from build123d import *

# Parameters (mm, degrees)
SKETCH1_R           = 15.75
SKETCH1_R_2         = 2
BOSS_EXTRUDE3_DEPTH = 10
SKETCH2_R           = 19.5
CUT_EXTRUDE1_DEPTH  = 10
CUT_EXTRUDE2_DEPTH  = 10
CUT_EXTRUDE3_DEPTH  = 10


with BuildPart() as part:
    # Sketch1 → Boss-Extrude3 (new body)
    with BuildSketch(Plane(origin=(0, 0, 0), x_dir=(1, 0, 0), z_dir=(0, 1, 0))):
        with BuildLine():
            Line((-52.326392464, -141.880675109), (47.673607536, -141.880675109))
            Line((47.673607536, -141.880675109), (47.673607536, 8.119324891))
            ThreePointArc((47.673607536, 8.119324891), (-2.326392464, 58.119324891), (-52.326392464, 8.119324891))
            Line((-52.326392464, 8.119324891), (-52.326392464, -141.880675109))
        make_face()
        with Locations((-2.326392464, 8.119324891)):
            Circle(SKETCH1_R, mode=Mode.SUBTRACT)
        with Locations((21.173607536, 8.119324891)):
            Circle(SKETCH1_R_2, mode=Mode.SUBTRACT)
        with Locations((9.423607536, -12.232272098)):
            Circle(SKETCH1_R_2, mode=Mode.SUBTRACT)
        with Locations((-14.076392464, -12.232272098)):
            Circle(SKETCH1_R_2, mode=Mode.SUBTRACT)
        with Locations((-25.826392464, 8.119324891)):
            Circle(SKETCH1_R_2, mode=Mode.SUBTRACT)
        with Locations((-14.076392464, 28.47092188)):
            Circle(SKETCH1_R_2, mode=Mode.SUBTRACT)
        with Locations((9.423607536, 28.47092188)):
            Circle(SKETCH1_R_2, mode=Mode.SUBTRACT)
        with Locations((-47.326392464, -116.880675109)):
            Circle(SKETCH1_R_2, mode=Mode.SUBTRACT)
        with Locations((42.673607536, -116.880675109)):
            Circle(SKETCH1_R_2, mode=Mode.SUBTRACT)
        with Locations((-37.326392464, -126.880675109)):
            Circle(SKETCH1_R_2, mode=Mode.SUBTRACT)
        with Locations((-37.326392464, -96.880675109)):
            Circle(SKETCH1_R_2, mode=Mode.SUBTRACT)
        with Locations((-47.326392464, -76.880675109)):
            Circle(SKETCH1_R_2, mode=Mode.SUBTRACT)
        with Locations((42.673607536, -76.880675109)):
            Circle(SKETCH1_R_2, mode=Mode.SUBTRACT)
        with Locations((-47.326392464, -56.880675109)):
            Circle(SKETCH1_R_2, mode=Mode.SUBTRACT)
        with Locations((42.673607536, -56.880675109)):
            Circle(SKETCH1_R_2, mode=Mode.SUBTRACT)
        with Locations((-27.326392464, -116.880675109)):
            Circle(SKETCH1_R_2, mode=Mode.SUBTRACT)
        with Locations((22.673607536, -116.880675109)):
            Circle(SKETCH1_R_2, mode=Mode.SUBTRACT)
        with Locations((-27.326392464, -56.880675109)):
            Circle(SKETCH1_R_2, mode=Mode.SUBTRACT)
        with Locations((-27.326392464, -76.880675109)):
            Circle(SKETCH1_R_2, mode=Mode.SUBTRACT)
        with Locations((22.673607536, -56.880675109)):
            Circle(SKETCH1_R_2, mode=Mode.SUBTRACT)
        with Locations((22.673607536, -76.880675109)):
            Circle(SKETCH1_R_2, mode=Mode.SUBTRACT)
        with Locations((32.673607536, -96.880675109)):
            Circle(SKETCH1_R_2, mode=Mode.SUBTRACT)
        with Locations((32.673607536, -126.880675109)):
            Circle(SKETCH1_R_2, mode=Mode.SUBTRACT)
    extrude(amount=BOSS_EXTRUDE3_DEPTH)

    # Sketch2 → Cut-Extrude1 (cut)
    with BuildSketch(Plane(origin=(0, 10, 0), x_dir=(1, 0, 0), z_dir=(0, 1, 0))):
        with Locations((-2.326392464, -96.880675109)):
            Circle(SKETCH2_R)
    extrude(amount=-CUT_EXTRUDE1_DEPTH, mode=Mode.SUBTRACT)

    # Sketch3 → Cut-Extrude2 (cut)
    with BuildSketch(Plane(origin=(0, 10, 0), x_dir=(1, 0, 0), z_dir=(0, 1, 0))):
        with BuildLine():
            Line((-7.326392464, -131.880675109), (-7.326392464, -115.728751934))
            ThreePointArc((-7.326392464, -115.728751934), (-2.326392464, -116.380675109), (2.673607536, -115.728751934))
            Line((2.673607536, -115.728751934), (2.673607536, -131.880675109))
            Line((2.673607536, -131.880675109), (-7.326392464, -131.880675109))
        make_face()
    extrude(amount=-CUT_EXTRUDE2_DEPTH, mode=Mode.SUBTRACT)

    # Sketch4 → Cut-Extrude3 (cut)
    with BuildSketch(Plane(origin=(0, 10, 0), x_dir=(1, 0, 0), z_dir=(0, 1, 0))):
        with BuildLine():
            ThreePointArc((-19.688674915, -88.003674033), (-16.114974697, -83.092092876), (-11.203393541, -79.518392659))
            Line((-11.203393541, -79.518392659), (-16.114974697, -74.606811502))
            Line((-16.114974697, -74.606811502), (-24.600256072, -83.092092876))
            Line((-24.600256072, -83.092092876), (-19.688674915, -88.003674033))
        make_face()
        with BuildLine():
            Line((11.462189769, -74.606811502), (6.550608612, -79.518392659))
            ThreePointArc((6.550608612, -79.518392659), (11.462189769, -83.092092876), (15.035889986, -88.003674033))
            Line((15.035889986, -88.003674033), (19.947471143, -83.092092876))
            Line((19.947471143, -83.092092876), (11.462189769, -74.606811502))
        make_face()
        with BuildLine():
            Line((19.947471143, -110.669257342), (15.035889986, -105.757676186))
            ThreePointArc((15.035889986, -105.757676186), (11.462189769, -110.669257342), (6.550608612, -114.24295756))
            Line((6.550608612, -114.24295756), (11.462189769, -119.154538717))
            Line((11.462189769, -119.154538717), (19.947471143, -110.669257342))
        make_face()
        with BuildLine():
            ThreePointArc((-11.203393541, -114.24295756), (-16.114974697, -110.669257342), (-19.688674915, -105.757676186))
            Line((-19.688674915, -105.757676186), (-24.600256072, -110.669257342))
            Line((-24.600256072, -110.669257342), (-16.114974697, -119.154538717))
            Line((-16.114974697, -119.154538717), (-11.203393541, -114.24295756))
        make_face()
    extrude(amount=-CUT_EXTRUDE3_DEPTH, mode=Mode.SUBTRACT)


solid = part.part
Build history of the part. All positions in model axes, mm. A direction names the side the tool comes from. Give positions to 0.01 mm unless a question says otherwise; leave off trailing zeros. Order: outer loops, then holes, each group sorted by start corner. A loop starts at its lowest first (then second) coordinate and runs counter-clockwise, first axis right, second up. Notation, with made-up numbers: M 7,-9 L 18,-9 A23 cw 18,14 Z; hole C -39,27.25 d8. An arc over 180 degrees is marked long. Put each result on its own line as item: value.
Item 1: Flat gauge pins, fed straight in: pin 1 Ø2.5 at (x, z) = (42.67, 56.88) entering from -Y; pin 2 Ø5 at (x, z) = (22.67, 116.88) entering from -Y. Where does each tip first touch, or does it go through?
From the geometry:
pin 1: passes through
pin 2: stops at y = 0
Item 2: Slice it at A-A, the plane z = 1. Write the cut outline in (x, y), plus the area to 3 significant figures.
From the geometry:
outline: M -52.33,0 L -15.17,0 L -15.17,10 L -52.33,10 Z; M 10.51,0 L 47.67,0 L 47.67,10 L 10.51,10 Z
area: 743 mm2
Item 3: Slice it at D-D, the plane y = 4.75. Give the number of separate pieces and of enclosed holes in the cut face, plus the area to 3 significant figures.
From the geometry:
separate pieces: 1
enclosed holes: 24
area: 16,200 mm2
Item 4: Two-plate mould, pull along Z, no slides. Class faces 1 (the flat face through (-3, 5, 141.881)), 2 (the cylindrical face through (-37.76, 4.93, 98.833)), 3 (the flat face through (47.674, 5, 68)): +Z half, -Z half, draft (parallel to the pull), parting line (faces both ways), or undercut.
From the geometry:
face 1: +Z half
face 2: undercut
face 3: draft
Item 5: Slice it at B-B, the plane x = -1. Write the cut outline in (y, z).
From the geometry:
outline: M 0,-58.1 L 10,-58.1 L 10,-23.81 L 0,-23.81 Z; M 0,7.57 L 10,7.57 L 10,77.43 L 0,77.43 Z; M 0,131.88 L 10,131.88 L 10,141.88 L 0,141.88 Z
Item 6: Probe line 1 (X direction, y = 7.25, z = 57); line 2 (Z direction, x = -39, y = 5.25); line 3 (Z direction, x = -9.5, y = 4.75). List the from-to ranges inside material, lowest first. Write a range as [from, to].
From the geometry:
line 1: x = [-52.33, -49.32], [-45.33, -29.32], [-25.33, 20.68], [24.67, 40.68], [44.67, 47.67]
line 2: z = [-42.11, 95.79], [97.98, 125.79], [127.98, 141.88]
line 3: z = [-57.6, -22.14], [5.9, 78.75], [115.01, 141.88]
Item 7: 3-axis set-ups, long thin cutter, end or side, ignore diameter. For faces 4 (the flat face through (-13.62, 5.07, 77.1)), 5 (the flat face through (-3, 0, 40)): which of +Z, -Z, +X, -X, +Y, -Y reach the whole face in a straight line?
From the geometry:
face 4: +Y, -Y
face 5: +Z, -Z, +X, -X, -Y
Item 8: Slice it at C-C, the plane z = 92.5. Write the cut outline in (x, y), plus the area to 3 significant figures.
From the geometry:
outline: M -52.33,0 L -21.33,0 L -21.33,10 L -52.33,10 Z; M 16.68,0 L 47.67,0 L 47.67,10 L 16.68,10 Z
area: 620 mm2
